from build123d import *

# Parameters (mm, degrees)
SKETCH1_R               = 70
BOSS_EXTRUDE1_DEPTH     = 3.5
BOSS_EXTRUDE2_DEPTH     = 12
M2_5_TAPPED_HOLE1_D     = 2.05
M2_5_TAPPED_HOLE1_DEPTH = 17
CUT_EXTRUDE4_START      = -12
CUT_EXTRUDE4_DEPTH      = 12


# Read off the part's stored shape, not the designer's step: CirPattern1
with BuildPart() as part:
    # Sketch1 → Boss-Extrude1 (new, symmetric)
    with BuildSketch(Plane.XY):
        Circle(SKETCH1_R)
    extrude(amount=BOSS_EXTRUDE1_DEPTH, both=True)

    # Sketch13 → Cut-Revolve1 (revolve, cut)
    with BuildSketch(Plane(origin=(0, 0, 0), x_dir=(0, 0, -1), z_dir=(1, 0, 0))):
        Polygon((-2.040406099, -59.376585203), (0.072455051, -70.377238659), (2.036555607, -70), (0.150362311, -60.17949722), align=None)
    revolve(axis=Axis((0, -70, 0), (0, 0.982050277997827, 0.18861932956192706)), mode=Mode.SUBTRACT)

    # CirPattern1 outline → CirPattern1 (revolve, cut)
    with BuildSketch(Plane(origin=(2.490740254, 0.009350069, 12.968088503), x_dir=(0, 1, 0), z_dir=(-0.188619329561927, 0, -0.982050277997827))):
        Polygon((0, 57.935114232), (2, 59.13683547), (2, 69.127313847), (0, 69.127313847), align=None)
    revolve(axis=Axis((2.490740254, 0.009350069, 12.968088503), (0.982050277997827, 0, -0.188619329561927)), mode=Mode.SUBTRACT)

    # CirPattern1 2 outline → CirPattern1 2 (revolve, cut)
    with BuildSketch(Plane(origin=(2e-08, 2.491072904, 12.969820451), x_dir=(1, 0, 0), z_dir=(0, 0.188619329561927, 0.982050277997827))):
        Polygon((0, 57.94429647), (2, 59.146017708), (2, 69.126976101), (0, 69.126976101), align=None)
    revolve(axis=Axis((2e-08, 2.491072904, 12.969820451), (0, 0.982050277997827, -0.188619329561927)), mode=Mode.SUBTRACT)

    # CirPattern1 3 outline → CirPattern1 3 (revolve, cut)
    with BuildSketch(Plane(origin=(-2.490740254, 0.009350089, 12.9680885), x_dir=(0, 1, 0), z_dir=(0.188619329561927, 0, -0.982050277997827))):
        Polygon((2, -69.127431112), (2, -59.136835451), (0, -57.935114213), (0, -69.127431112), align=None)
    revolve(axis=Axis((-2.490740254, 0.009350089, 12.9680885), (0.982050277997827, 0, 0.188619329561927)), mode=Mode.SUBTRACT)

    # Sketch4 → Boss-Extrude2 (add)
    with BuildSketch(Plane(origin=(0, 0, -3.5), x_dir=(-1, 0, 0), z_dir=(0, 0, -1))):
        Polygon((31.875552268, 8.541028488), (48.296291314, 12.940952255), (45.708100863, 22.600210518), (40.878471732, 21.306115293), (42.690205048, 14.544634508), (31.099095132, 11.438805967), align=None)
        Polygon((56.785555994, -18.741414847), (51.955926862, -20.035510073), (50.144193547, -13.274029289), (38.553083631, -16.37985783), (37.776626496, -13.482080351), (54.197365543, -9.082156584), align=None)
    boss_extrude2 = extrude(amount=BOSS_EXTRUDE2_DEPTH)

    # M2.5 Tapped Hole1
    with Locations(Plane(origin=(-48.296291314, 12.940952255, 0), x_dir=(0, 0, 1), z_dir=(-0.9659258262890691, 0.2588190451025179, 0))):
        with Locations((-9.7, 2.35), (-9.7, -25.15)):
            m2_5_tapped_hole1 = Hole(M2_5_TAPPED_HOLE1_D / 2, depth=M2_5_TAPPED_HOLE1_DEPTH)

    # Mirror1: Boss-Extrude2, M2.5 Tapped Hole1 across plane
    add(boss_extrude2.mirror(Plane(origin=(0, 0, 0), x_dir=(0, 0, 1), z_dir=(1, 0, 0))))
    add(m2_5_tapped_hole1.mirror(Plane(origin=(0, 0, 0), x_dir=(0, 0, 1), z_dir=(1, 0, 0))), mode=Mode.SUBTRACT)

    # Sketch7 → Cut-Extrude4 (cut)
    with BuildSketch(Plane(origin=(0, 0, -3.5), x_dir=(-1, 0, 0), z_dir=(0, 0, -1)).offset(CUT_EXTRUDE4_START)):
        with BuildLine():
            ThreePointArc((-57.113972469, -40.472140403), (-41.814961007, -44.896509701), (-36.315733397, -59.842856782))
            ThreePointArc((-36.315733397, -59.842856782), (-47.708318434, -51.224177419), (-57.113972469, -40.472140403))
        make_face()
    extrude(amount=CUT_EXTRUDE4_DEPTH, mode=Mode.SUBTRACT)


solid = part.part
Model file for the job. Use its own axes, mm. A direction names the side the tool comes from. Give positions to 0.01 mm unless a question says otherwise; leave off trailing zeros. Write each loop counter-clockwise with the first axis right and the second up, starting at its lowest first coordinate (ties: lowest second). Pieces come first, ordered by that corner, then holes. Notation, with made-up numbers: (25, 77) - (65, 77) arc R11 cw to (65, 92) - close; hole circle Ø9 at (-29.75, 83). An arc over 180 degrees is marked (long way). Answer as CSV lines item,"result".
1. Band-saw the part on A-A (x = -9). Write the cut outline in (y, z), and give its area (3 significant figures).
Responses:
outline,"(-69.42, -3.5) - (69.42, -3.5) - (69.42, 3.5) - (-69.42, 3.5) - close"
area,"972 mm2"
2. Drill centre lines: L1, parallel to Z at x = 22.5, y = 17.5; L2, parallel to X at y = -63, z = 2; L3, parallel to X at y = 34.5, z = -2.75. Where is each one in solid material? Low to high. Write a range as [from, to].
Responses:
L1,"z = [-3.5, 3.5]"
L2,"x = [-30.51, -1.89], [1.89, 30.51]"
L3,"x = [-60.91, 60.91]"
3. Two-plate mould, pull along Z, no slides. Class faces 5 (the face through (-51.063, -16.702, -9.416)), 6 (the face through (46.2, -12.6, -9.6)), 7 (the face through (43, 15, -15.5)): +Z half, -Z half, draft (parallel to the pull), parting line (faces both ways), or undercut.
Responses:
face 5,"draft"
face 6,"undercut"
face 7,"-Z half"
4. Pin check, flat tips, straight feed: pin 1 (4 mm diameter, centred on x = -33.5, y = -5, fed in from -Z); pin 2 (6 mm diameter, centred on y = 42.5, z = -2, fed in from +X); pin 3 (8 mm diameter, centred on x = -32, z = -12, fed in from -Y). Stop position of each tip, or through.
Responses:
pin 1,"stops at z = -3.5"
pin 2,"stops at x = 57.79"
pin 3,"stops at y = 8.54"
5. Band-saw the part on B-B (y = -57.5). Write the cut outline in (x, z), and give its area (3 significant figures).
Responses:
outline,"(-39.92, -3.5) - (36.2, -3.5) - (36.2, 3.5) - (-39.92, 3.5) - close"
area,"533 mm2"
6. 3-axis set-ups, long thin cutter, end or side, ignore diameter. For faces 1 (the face through (45.872, -11.313, -9.416)), 2 (the face through (-0.045, 59.535, 1.663)), 3 (the face through (-44.43, -14.805, -6.166)), 4 (the face through (-54.4, -19.38, -9.42)): which of +Z, -Z, +X, -X, +Y, -Y reach the whole face in a straight line?
Responses:
face 1,"-Z"
face 2,"none"
face 3,"-Z, -Y"
face 4,"-Z, -X, -Y"
